Source: CAD feature listing. Evaluate the final solid. Frame: model axes, mm. Coordinates: 2 decimals unless noted, no trailing zeros. Loops run counter-clockwise (first coordinate to the right, second up) from the corner with the lowest first, then second, coordinate; pieces in that order, holes last.
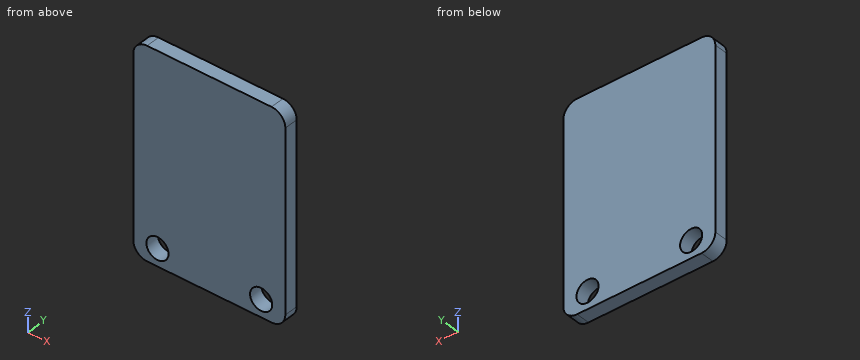
Autodesk Inventor part; units mm, degrees
ref_plane "YZ Plane" through (0, 0, 0) normal (1, 0, 0) x (0, 1, 0)
ref_plane "XZ Plane" through (0, 0, 0) normal (0, 1, 0) x (-1, 0, 0)
ref_plane "XY Plane" through (0, 0, 0) normal (0, 0, 1) x (1, 0, 0)
sketch "Esquisse1" plane through (0, 0, 0) normal (0, 1, 0) x (-1, 0, 0)
  line L0 (0, 0) -> (22, 0)
  line L1 (22, 0) -> (22, -30)
  line L2 (22, -30) -> (0, -30)
  line L3 (0, -30) -> (0, 0)
  dimension "d0" = 22
  dimension "d1" = 30
extrude "Extrusion1" add sketch "Esquisse1" along normal blind 2
sketch "Esquisse2" plane through (0, 2, 0) normal (0, 1, 0) x (1, 0, 0)
  line L0 (0, 30) -> (-22, 30)
  line L1 (-11, 30) -> (-3.5, 30)
  line L2 (-11, 30) -> (-18.5, 30)
  line L3 (-18.5, 30) -> (-18.5, 27.5)
  line L4 (-3.5, 30) -> (-3.5, 27.5)
  circle A0 centre (-18.5, 27.5) radius 1.6
  circle A1 centre (-3.5, 27.5) radius 1.6
  point P0 (0, 0)
  dimension "d4" = 7.5
  dimension "d5" = 7.5
  dimension "d6" = 2.5
  dimension "d7" = 2.5
  dimension "d8" = 3.2
  dimension "d9" = 3.2
extrude "Extrusion2" cut sketch "Esquisse2" against normal through all
fillet "Congé1" radius 2 4 edges at (0, 1, -30) (-22, 1, -30) (0, 1, 0) (-22, 1, 0)
properties part number "DFR0440"
Q1. Section C-C, the plane y = 1.35. Return the cut outline in (x, z), plus the area to 3 significant figures.
Q2. Section B-B, the plane z = -27.5. Return the cut outline in (x, y).
Q3. Section D-D, the plane x = -2.75. Return the cut outline in (y, z).
Q4. Line query: line 1 along X through (y, z) = (1.25, -27.5); line 2 along Z through (x, y) = (-18.5, 1.1); line 3 along Z through (x, y) = (-2.75, 0.45). Output: solid intervals per line, ascending.
Q5. Section A-A, the plane x = -18.5. Return the cut outline in (y, z), plus the area to 3 significant figures.
Derived:
1. outline: (-22, -28) arc R2 ccw to (-20, -30) - (-2, -30) arc R2 ccw to (0, -28) - (0, -2) arc R2 ccw to (-2, 0) - (-20, 0) arc R2 ccw to (-22, -2) - close; hole circle Ø3.2 at (-18.5, -27.5); hole circle Ø3.2 at (-3.5, -27.5)
1. area: 640 mm2
2. outline: (-22, 0) - (-20.1, 0) - (-20.1, 2) - (-22, 2) - close; (-16.9, 0) - (-5.1, 0) - (-5.1, 2) - (-16.9, 2) - close; (-1.9, 0) - (0, 0) - (0, 2) - (-1.9, 2) - close
3. outline: (0, -30) - (2, -30) - (2, -28.91) - (0, -28.91) - close; (0, -26.09) - (2, -26.09) - (2, 0) - (0, 0) - close
4. line 1: x = -22 to -20.1, -16.9 to -5.1, -1.9 to 0
4. line 2: z = -30 to -29.1, -25.9 to 0
4. line 3: z = -30 to -28.91, -26.09 to 0
5. outline: (0, -30) - (2, -30) - (2, -29.1) - (0, -29.1) - close; (0, -25.9) - (2, -25.9) - (2, 0) - (0, 0) - close
5. area: 53.6 mm2
